For this review, use the dimensioned drawing (mm, ordinates from the lowest corner) and the shaded views. A direction names the side the tool comes from. Coordinates: 2 decimals unless noted, no trailing zeros. Loops run counter-clockwise (first coordinate to the right, second up) from the corner with the lowest first, then second, coordinate; pieces in that order, holes last. Notation, with made-up numbers: (32.5, 9) -> (74.5, 9) arc R19 cw to (74.5, 41) -> close; hole circle Ø9 at (-10.5, 25). An arc over 180 degrees is marked (long way). Answer as a JSON object with one key per item and string values.
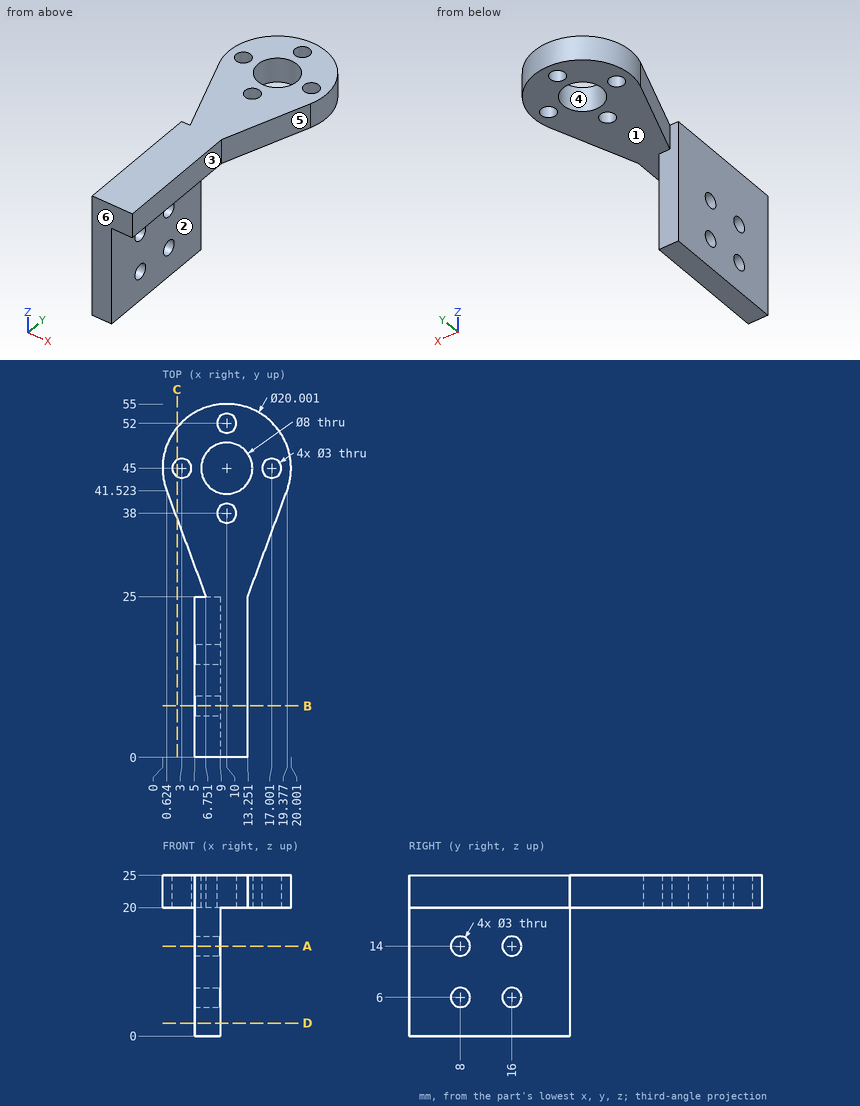
1) Clearance check with flat-ended pins moving along their axes: pin 1 Ø4 at (y, z) = (16, 14) entering from -X; pin 2 Ø1.8 at (y, z) = (16, 6) entering from -X; pin 3 Ø1.5 at (y, z) = (16.5, 23) entering from +X; pin 4 Ø5 at (x, z) = (13, 18) entering from +Y. State where each tip first meets the part, or that it passes through.
Completed:
{"pin 1": "x = 5", "pin 2": "through", "pin 3": "x = 13.25", "pin 4": "y = 54.89"}
2) The part is to be moulded in two halves that separate along X. For the marked faces 4, 5 and 6, say which applies: pulls with the +X half, pulls with the -X half, needs draft (parallel to the pull), parting line crosses it, or undercut.
Completed:
{"face 4": "undercut", "face 5": "pulls with the +X half", "face 6": "needs draft"}
3) Add section D-D, the plane z = 2. Give the boundary of the cut face in (x, y), and give its area (3 significant figures).
Completed:
{"outline": "(5, 0) -> (9, 0) -> (9, 25) -> (5, 25) -> close", "area": "100 mm²"}
4) Add section A-A, the plane z = 14. Give the boundary of the cut face in (x, y).
Completed:
{"outline": "(5, 0) -> (9, 0) -> (9, 6.5) -> (5, 6.5) -> close; (5, 9.5) -> (9, 9.5) -> (9, 14.5) -> (5, 14.5) -> close; (5, 17.5) -> (9, 17.5) -> (9, 25) -> (5, 25) -> close"}
5) Add section B-B, the plane y = 8. Give the boundary of the cut face in (x, z).
Completed:
{"outline": "(5, 0) -> (9, 0) -> (9, 4.5) -> (5, 4.5) -> close; (5, 7.5) -> (9, 7.5) -> (9, 12.5) -> (5, 12.5) -> close; (5, 15.5) -> (9, 15.5) -> (9, 20) -> (13.25, 20) -> (13.25, 25) -> (5, 25) -> close"}
6) Wall thickness on probe 1 along Z at (x, y) = (8.05, 16); probe 2 along X at (y, z) = (21, 3.5); probe 3 along Z at (x, y) = (6, 41): over which ranges is each line inside the solid? List them lowest first.
Completed:
{"probe 1": "0 to 4.5, 7.5 to 12.5, 15.5 to 25", "probe 2": "5 to 9", "probe 3": "20 to 25"}
7) For the marked faces 1, 2 and 3, list the 3-axis set-ups (+Z, -Z, +X, -X, +Y, -Y) from which the entire face can be reached by the end or side of a thin tool; tool diameter is ignored.
Completed:
{"face 1": "-Z, +X, +Y", "face 2": "-Z, +X, +Y, -Y", "face 3": "+Z, -Z, +X, -Y"}
8) Add section C-C, the plane x = 2.25. Give the boundary of the cut face in (y, z).
Completed:
{"outline": "(37.14, 20) -> (43.7, 20) -> (43.7, 25) -> (37.14, 25) -> close; (46.3, 20) -> (51.32, 20) -> (51.32, 25) -> (46.3, 25) -> close"}
